Here's how the part is built. I have some questions about the finished solid (model axes, mm). A direction names the side the tool comes from. Round coordinates to 2 decimals unless told otherwise and drop trailing zeros. Loops run counter-clockwise (first coordinate to the right, second up) from the corner with the lowest first, then second, coordinate; pieces in that order, holes last. Notation, with made-up numbers: (-5.75, 43) -> (50.25, 43) arc R21 cw to (50.25, 48) -> close; hole circle Ø7 at (56.25, 43). An arc over 180 degrees is marked (long way). Use CSV: the item, a comma, the result in double quotes. Start each with the question number.
from build123d import *

# Parameters (mm, degrees)
EXTRUDE_1_DEPTH              = 8
HOLE_WIZARD_M4_1_D           = 3.3
HOLE_WIZARD_M4_1_DEPTH       = 5
HOLE_WIZARD_M4_1_CSINK_D     = 4.05
HOLE_WIZARD_M4_1_CSINK_ANGLE = 90
HOLE_WIZARD_M4_1_TIP         = 0.991420021
MOVE_BODY_1_ANGLE            = 90


# Read off the part's stored shape, not the designer's step: M4 机械螺纹 螺柱1
with BuildPart() as part:
    # 草图1 → 凸台-拉伸1 (new body)
    with BuildSketch(Plane.XY):
        Polygon((3.464101615, 0), (1.732050808, 3), (-1.732050808, 3), (-3.464101615, 0), (-1.732050808, -3), (1.732050808, -3), align=None)
    extrude(amount=EXTRUDE_1_DEPTH)

    # M4 螺纹孔1
    with Locations(Plane(origin=(0, 0, 0), x_dir=(-1, 0, 0), z_dir=(0, 0, -1))):
        with Locations((0, 0)):
            CounterSinkHole(HOLE_WIZARD_M4_1_D / 2, HOLE_WIZARD_M4_1_CSINK_D / 2, depth=HOLE_WIZARD_M4_1_DEPTH, counter_sink_angle=HOLE_WIZARD_M4_1_CSINK_ANGLE)
            with Locations((0, 0, -(HOLE_WIZARD_M4_1_DEPTH + HOLE_WIZARD_M4_1_TIP / 2))):  # 118° drill point
                Cone(0, HOLE_WIZARD_M4_1_D / 2, HOLE_WIZARD_M4_1_TIP, mode=Mode.SUBTRACT)

    # M4 机械螺纹 螺柱1 outline → M4 机械螺纹 螺柱1 (revolve)
    with BuildSketch(Plane.XZ):
        Polygon((1.621, 15), (0, 15), (0, 8), (2, 8), (2, 14.621), align=None)
    revolve(axis=Axis((0, 0, 0), (0, 0, 1)))


with BuildPart() as part_1:
    # Move Body 1: moved
    add(part.part.rotate(Axis((0, 0, 6), (-1, 0, 0)), MOVE_BODY_1_ANGLE))


solid = part_1.part
Q1. Will this pin go through, and if not, where does the flat tip stop? pin 1 Ø1.5 at (x, y) = (-0.5, 4.5) entering from +Z.
Q2. If we mould it in two halves opening along Z, with no side actions, what happens to faces 1 (the flat face through (-2.6, -2.1, 4.5)), 2 (the flat face through (1, 2, 4)), 3 (the conical face through (0.21, -0.18, 5.81)), 4 (the cylindrical face through (0, 5, 8))? For each: pulls with the +Z half, pulls with the -Z half, needs draft (parallel to the pull), parting line crosses it, or undercut.
Q3. I need wall thicknesses on line 1 along Z through (x, y) = (0, -3.8); line 2 along Y through (x, z) = (3, 5.25); line 3 along Z through (x, y) = (0.5, 4.5). Which ranges of each line are inside material? Lowest first, please.
Q4. I want a section at A-A, the plane y = -1.5. List the corners of the cut face in (x, z) for me, then the cut area to 3 significant figures.
Q5. For faces 5 (the flat face through (2.6, -2.1, 4.5)), 6 (the cylindrical face through (-0.4, -3.3, 7.6)), which set-ups out of +Z, -Z, +X, -X, +Y, -Y let a thin tool reach every point of the face, with its end or its side?
Q6. I want a section at B-B, the plane y = 8. List the corners of the cut face in (x, z) for me, then the cut area to 3 significant figures.
Values found:
1,pin 1,"z = 8"
2,face 1,"pulls with the -Z half"
2,face 2,"needs draft"
2,face 3,"undercut"
2,face 4,"parting line crosses it"
3,line 1,"3 to 4.35, 7.65 to 9"
3,line 2,"-6 to 2"
3,line 3,"4.06 to 7.94"
4,outline,"(-3.46, 6) -> (-1.73, 3) -> (1.73, 3) -> (3.46, 6) -> (1.73, 9) -> (-1.73, 9) -> close; hole circle Ø3.3 at (0, 6)"
4,area,"22.6 mm2"
5,face 5,"-Z, +X, +Y, -Y"
5,face 6,"-Y"
6,outline,"circle Ø4 at (0, 6)"
6,area,"12.6 mm2"
